Verification items for the finished model (mm, model axes). Coordinates: 2 decimals unless noted, no trailing zeros. Loops run counter-clockwise (first coordinate to the right, second up) from the corner with the lowest first, then second, coordinate; pieces in that order, holes last.
Q1. Sectioned sample at B-B (x = 458). Enter the section's corners in (y, z) (3 decimals), then the cut area to 3 significant figures.
Q2. Material ranges on probe 1 along X at (y, z) = (-201.5, 0.55); probe 2 along Y at (x, z) = (338, 0.5); probe 3 along Y at (x, z) = (727, 0.6), recorded low to high.
Q3. Go/stop test with flat-tipped pins: P1, Ø1, axis at y = 35, z = 1, coming from the +X side; P2, Ø1.5, axis at y = 35.5, z = 1, coming from the -X side. Record where each tip stops, or that it passes through.
Q4. Sectioned sample at A-A (x = 333). Enter the section's corners in (y, z) (3 decimals), then the cut area to 3 significant figures.
```python
from build123d import *

# Parameters (mm, degrees)
BOSS_EXTRUDE1_DEPTH = 3.175


with BuildPart() as part:
    # Sketch1 → Boss-Extrude1 (new body)
    with BuildSketch(Plane.XY):
        with BuildLine():
            Line((771.903793001, 164.465805668), (771.903793001, 186.055805664))
            Line((771.903793001, 186.055805664), (654.555793001, 186.055805664))
            ThreePointArc((654.555793001, 186.055805664), (593.014276043, 157.121992999), (558.8, 98.352042006))
            ThreePointArc((558.8, 98.352042006), (462.094129135, -80.619143391), (287.082829619, -184.319460189))
            ThreePointArc((287.082829619, -184.319460189), (260.024944938, -202.483344486), (249.571639661, -233.350547549))
            Line((249.571639661, -233.350547549), (249.571639661, -266.960111933))
            ThreePointArc((249.571639661, -266.960111933), (251.803485989, -272.348265606), (257.191639661, -274.580111933))
            Line((257.191639661, -274.580111933), (372.702998231, -274.580111933))
            ThreePointArc((372.702998231, -274.580111933), (501.162126515, -221.370598787), (554.371639661, -92.911470503))
            add(Edge.make_bspline(
                [(554.371639661, -92.911470503), (554.371639661, 52.307938416), (646.172603674, 136.193906474), (771.903793001, 164.465805668)],
                knots=[0, 0, 0, 0, 1, 1, 1, 1], degree=3))
        make_face()
    extrude(amount=BOSS_EXTRUDE1_DEPTH)


solid = part.part
```
Geometry check:
1. outline: (-253.311, 0) - (-84.813, 0) - (-84.813, 3.175) - (-253.311, 3.175) - close
1. area: 535 mm2
2. probe 1: x = 260.8 to 518.35
2. probe 2: y = -274.58 to -166.57
2. probe 3: y = 151.44 to 186.06
3. P1: stops at x = 584.65
3. P2: stops at x = 538.22
4. outline: (-274.58, 0) - (-168.675, 0) - (-168.675, 3.175) - (-274.58, 3.175) - close
4. area: 336 mm2
